Check sheet for the drawn part. Datum: minimum x, y, z corner. Units: mm. Give positions to 0.01 mm unless a question says otherwise; leave off trailing zeros. Loops run counter-clockwise (first coordinate to the right, second up) from the corner with the lowest first, then second, coordinate; pieces in that order, holes last. Notation, with made-up numbers: (20.25, -29) - (49.25, -29) arc R18 cw to (49.25, -18) - close; hole circle Ø2 at (28.5, 60). An arc over 180 degrees is marked (long way). Answer in a Markdown table with one row per item.
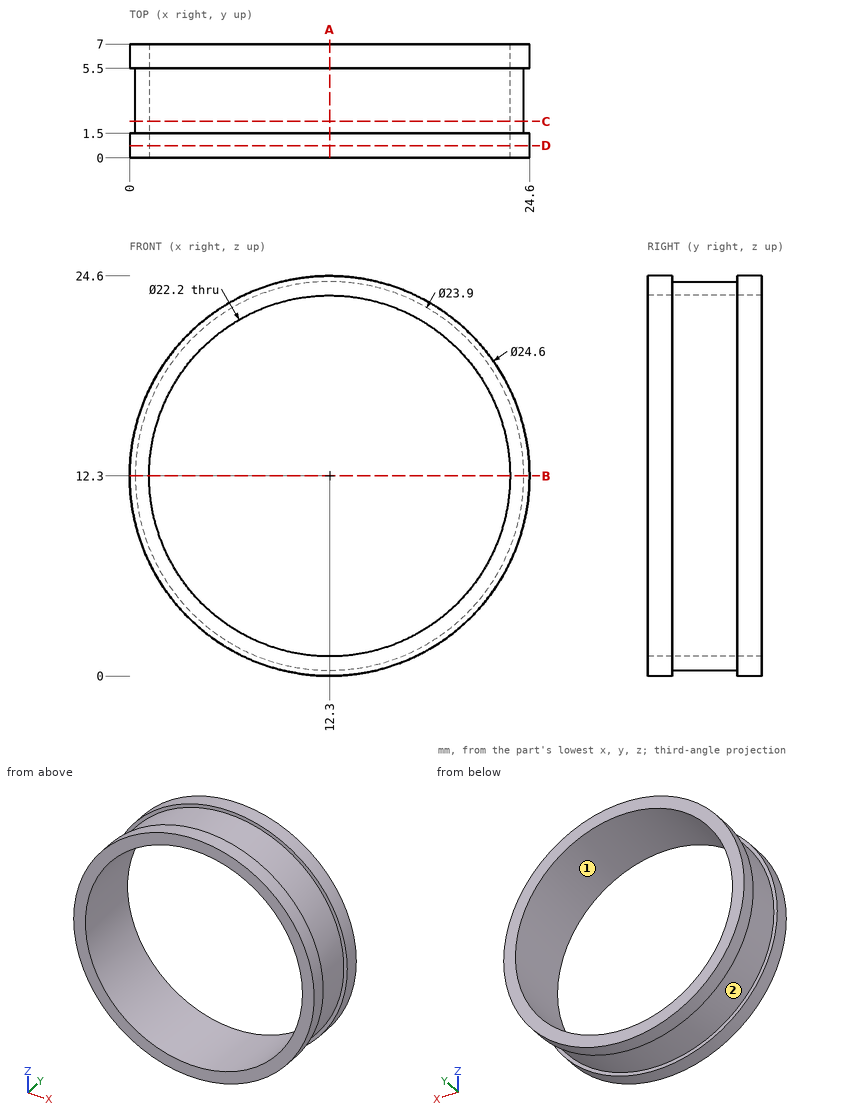
Q1. Sectioned sample at D-D (y = 0.75). Record the cut outline in (x, z).
Completed:
| item | result |
|---|---|
| outline | circle Ø24.6 at (12.3, 12.3); hole circle Ø22.2 at (12.3, 12.3) |
Q2. Sectioned sample at B-B (z = 12.3). Record the cut outline in (x, y).
Completed:
| item | result |
|---|---|
| outline | (0, 0) - (1.2, 0) - (1.2, 7) - (0, 7) - (0, 5.5) - (0.35, 5.5) - (0.35, 1.5) - (0, 1.5) - close; (23.4, 0) - (24.6, 0) - (24.6, 1.5) - (24.25, 1.5) - (24.25, 5.5) - (24.6, 5.5) - (24.6, 7) - (23.4, 7) - close |
Q3. Thickness scan on line 1 (Z direction, x = 12.3, y = 2.5); line 2 (Z direction, x = 3.5, y = 3.5); line 3 (X direction, y = 0.5, z = 22.5). Record the ranges inside material, lowest first.
Completed:
| item | result |
|---|---|
| line 1 | 0.35 to 1.2, 23.4 to 24.25 |
| line 2 | 4.22 to 5.53, 19.07 to 20.38 |
| line 3 | 5.43 to 7.92, 16.68 to 19.17 |
Q4. Draft check along Z on the marked faces 1 and 2. Enter one of: +Z half, -Z half, draft (parallel to the pull), parting line (faces both ways), or undercut.
Completed:
| item | result |
|---|---|
| face 1 | undercut |
| face 2 | parting line |
Q5. Sectioned sample at C-C (y = 2.25). Record the cut outline in (x, z).
Completed:
| item | result |
|---|---|
| outline | circle Ø23.9 at (12.3, 12.3); hole circle Ø22.2 at (12.3, 12.3) |
Q6. Sectioned sample at A-A (x = 12.3). Record the cut outline in (y, z), and give its area (3 significant figures).
Completed:
| item | result |
|---|---|
| outline | (0, 0) - (1.5, 0) - (1.5, 0.35) - (5.5, 0.35) - (5.5, 0) - (7, 0) - (7, 1.2) - (0, 1.2) - close; (0, 23.4) - (7, 23.4) - (7, 24.6) - (5.5, 24.6) - (5.5, 24.25) - (1.5, 24.25) - (1.5, 24.6) - (0, 24.6) - close |
| area | 14.0 mm^2 |
Q7. Go/stop test with flat-tipped pins: P1, Ø4, axis at y = 6, z = 16, coming from the -X side; P2, Ø3, axis at x = 14, y = 4.5, coming from the +Z side; P3, Ø3, axis at x = 3, y = 3.5, coming from the -Z side. Record where each tip stops, or that it passes through.
Completed:
| item | result |
|---|---|
| P1 | x = 0.12 |
| P2 | z = 24.59 |
| P3 | z = 3.25 |
